Check sheet for the modelled part. Datum: model origin and axes. Units: mm. Give positions to 0.01 mm unless a question says otherwise; leave off trailing zeros. Write each loop counter-clockwise with the first axis right and the second up, starting at its lowest first coordinate (ties: lowest second). Pieces come first, ordered by that corner, then holes. Notation, with made-up numbers: M 3,31.25 L 26,31.25 A33 cw 26,69.25 Z; hole C 47.5,-7 d10. An arc over 180 degrees is marked long. Use CSV: the item, a comma, the result in double quotes. Start each with the question number.
1. Depth check by flat-ended pin: P1, Ø2.5, axis at y = 3, z = 93.5, coming from the -X side; P2, Ø1.5, axis at x = -49, y = 2.5, coming from the +Z side; P3, Ø1.5, axis at y = 2.5, z = 92.5, coming from the +X side. Enter the tip coordinate at first touch or a pass-through.
2. Cross-section at B-B, the plane x = 65. Enter the section's corners in (y, z), and give its area (3 significant figures).
3. Scan lines: line 1 (Z direction, x = -6.5, y = 0.6); line 2 (X direction, y = 4.7, z = 93); line 3 (Z direction, x = 47.5, y = 3.1). Record each from-to range of solid material in increasing order.
4. Cross-section at A-A, the plane y = 3.9. Enter the section's corners in (x, z), and give its area (3 significant figures).
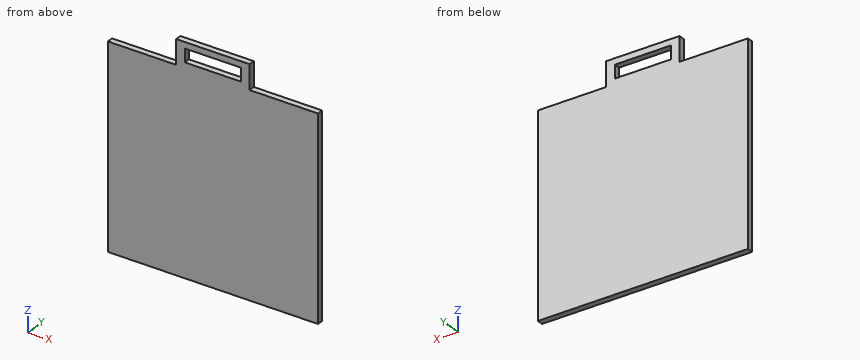
Autodesk Inventor part; units mm, degrees
ref_plane "YZ Plane" through (0, 0, 0) normal (1, 0, 0) x (0, 1, 0)
ref_plane "XZ Plane" through (0, 0, 0) normal (0, 1, 0) x (-1, 0, 0)
ref_plane "XY Plane" through (0, 0, 0) normal (0, 0, 1) x (1, 0, 0)
sketch "Sketch1" plane through (0, 0, 0) normal (0, 1, 0) x (-1, 0, 0)
  line L0 (120.4, 0) -> (-120.4, 0)
  line L1 (0, -117.6) -> (0, 117.6)
  line L2 (-86, 84) -> (86, 84)
  line L3 (86, 84) -> (86, -84)
  line L4 (86, -84) -> (-86, -84)
  line L5 (-86, -84) -> (-86, 84)
  line L6 (-86, 84) -> (86, -84) construction
  line L7 (86, 84) -> (-86, -84) construction
  point P0 (0, 0)
  dimension "d0" = 172
  dimension "d1" = 168
extrude "Extrusion1" add sketch "Sketch1" along normal blind 9
sketch "Sketch2" plane through (-86, 0, 84) normal (0, 0, 1) x (1, 0, 0)
  line L0 (172, 9) -> (0, 9)
  line L1 (172, 0) -> (0, 0)
  line L2 (56, 9) -> (116, 9)
  line L3 (116, 9) -> (116, 0)
  line L4 (116, 0) -> (56, 0)
  line L5 (56, 0) -> (56, 9)
  point P0 (86, 0)
  dimension "d4" = 60
  dimension "d5" = 30
extrude "Extrusion2" add sketch "Sketch2" along normal blind 20
sketch "Sketch3" plane through (0, 9, 0) normal (0, 1, 0) x (1, 0, 0)
  line L0 (-23, -88.1983) -> (23, -88.1983)
  line L1 (23, -88.1983) -> (23, -99)
  line L2 (23, -99) -> (-23, -99)
  line L3 (-23, -99) -> (-23, -88.1983)
  line L4 (30, -84) -> (30, -104)
  line L5 (30, -104) -> (-30, -104)
  line L6 (-30, -84) -> (-30, -104)
  line L7 (30, -84) -> (86, -84)
  point P0 (0, 0)
  dimension "d8" = 7
  dimension "d9" = 5
  dimension "d10" = 7
  dimension "d11" = 4.1983
extrude "Extrusion3" cut sketch "Sketch3" against normal blind 20
move faces "Move1" translate (0, -4, 0) faces at (-10, 9, -28)
move faces "Move2" translate (0, 0, 5) faces at (28.6667, 1.6667, -84)
properties part number "pokrywa"
Worked answers:
1,P1,"stops at x = -30"
1,P2,"stops at z = 84"
1,P3,"stops at x = 30"
2,outline,"M 0,-79 L 5,-79 L 5,84 L 0,84 Z"
2,area,"815 mm^2"
3,line 1,"z = -79 to 88.2, 99 to 104"
3,line 2,"x = -30 to -23, 23 to 30"
3,line 3,"z = -79 to 84"
4,outline,"M -86,-79 L 86,-79 L 86,84 L 30,84 L 30,104 L -30,104 L -30,84 L -86,84 Z; hole M -23,88.2 L 23,88.2 L 23,99 L -23,99 Z"
4,area,"28,700 mm^2"
